The listing builds one solid part. Answer for the finished solid, in the listing's coordinates (mm). Round coordinates to 2 decimals unless told otherwise and drop trailing zeros.
(1) The mould has two halves that part along Z. Classify faces 1 (the face through (7, 7, 0)), 2 (the face through (15, 7, -99)), 3 (the face through (7.4, 7.43, -193.45)), 4 (the face through (7, 8, -200)): +Z half, -Z half, draft (parallel to the pull), parting line (faces both ways), or undercut.
(2) This flat-tipped pin is pushed along its axis until it touches: pin 1 Ø1.9 at (y, z) = (7.5, -45) entering from +X. Where does it stop, or does it pass through?
(3) Find the intervals of material crossed by probe 1 along Z at (x, y) = (11.5, 7.5); probe 2 along X at (y, z) = (11.75, -185); probe 3 along Z at (x, y) = (7.5, 8.5), in increasing order.
Autodesk Inventor part; units mm, degrees
ref_plane "YZ Plane" through (0, 0, 0) normal (1, 0, 0) x (0, 1, 0)
ref_plane "XZ Plane" through (0, 0, 0) normal (0, 1, 0) x (-1, 0, 0)
ref_plane "XY Plane" through (0, 0, 0) normal (0, 0, 1) x (1, 0, 0)
sketch "スケッチ1" plane through (0, 0, 0) normal (1, 0, 0) x (0, 1, 0)
  line L0 (0, 0) -> (15, 0)
  line L1 (15, 0) -> (15, -200)
  line L2 (15, -200) -> (0, -200)
  line L3 (0, -200) -> (0, 0)
  dimension "d0" = 15
  dimension "d1" = 200
extrude "押し出し1" add sketch "スケッチ1" along normal blind 15
sketch "スケッチ2" plane through (15, 0, 0) normal (1, 0, 0) x (0, 0, -1)
  line L0 (200, 0) -> (200, 15)
  line L1 (0, 15) -> (0, 0)
  point P0 (195, 7.5)
  point P1 (45, 7.5)
  point P2 (200, 7.5)
  point P3 (200, 7.5)
  point P4 (200, 7.5)
  point P5 (0, 7.5)
  dimension "d4" = 5
  dimension "d5" = 45
hole "穴1" at (15, 7.5, -195) at (15, 7.5, -45) direction (-1, 0, 0) diameter 3.1 end through all
sketch "スケッチ3" plane through (0, 15, 0) normal (0, 1, 0) x (1, 0, 0)
  line L0 (0, 200) -> (15, 200)
  point P0 (0, 0)
  point P1 (7.5, 185)
  point P2 (7.5, 200)
  point P3 (7.5, 200)
  dimension "d13" = 15
hole "穴2" at (7.5, 15, -185) direction (0, -1, 0) diameter 3.1 end through all
properties part number "Dai"
Solutions:
1. face 1: +Z half
1. face 2: draft
1. face 3: undercut
1. face 4: -Z half
2. pin 1: passes through
3. probe 1: z = -200 to -196.55, -193.45 to -46.55, -43.45 to 0
3. probe 2: x = 0 to 5.95, 9.05 to 15
3. probe 3: z = -200 to -196.18, -193.82 to -186.55, -183.45 to -46.18, -43.82 to 0
